```python
from build123d import *

# Parameters (mm, degrees)
SKETCH_W        = 105
SKETCH_H        = 110
PAD_DEPTH       = 7.5
SKETCH001_R     = 1.25
POCKET_DEPTH    = 8
SKETCH002_R     = 3
POCKET001_DEPTH = 6
SKETCH003_W     = 85
SKETCH003_H     = 110
SKETCH003_W_2   = 81
SKETCH003_H_2   = 106
PAD001_DEPTH    = 57
SKETCH004_R     = 3.29
POCKET002_DEPTH = 6
SKETCH005_W     = 10
SKETCH005_H     = 110
POCKET003_DEPTH = 4
SKETCH006_W     = 10
SKETCH006_H     = 110
POCKET004_DEPTH = 4
SKETCH007_R     = 2.5
POCKET005_DEPTH = 5
SKETCH008_W     = 16
SKETCH008_H     = 16
POCKET006_DEPTH = 5
SKETCH009_R     = 1.25
SKETCH009_W     = 3.5
SKETCH009_H     = 7.5
POCKET007_DEPTH = 5


with BuildPart() as part:
    # Sketch → Pad (new body)
    with BuildSketch(Plane.XY):
        Rectangle(SKETCH_W, SKETCH_H)
    extrude(amount=PAD_DEPTH)

    # Sketch001 (on Face6 of Pad) → Pocket (cut)
    with BuildSketch(Plane.XY.offset(7.5)):
        with Locations((-33.5, 41.5)):
            Circle(SKETCH001_R)
        with Locations((15.5, 41.5)):
            Circle(SKETCH001_R)
        with Locations((-33.5, -16.5)):
            Circle(SKETCH001_R)
        with Locations((15.5, -16.5)):
            Circle(SKETCH001_R)
    extrude(amount=-POCKET_DEPTH, mode=Mode.SUBTRACT)

    # Sketch002 (on Face4 of Pocket) → Pocket001 (cut)
    with BuildSketch(Plane(origin=(0, 0, 0), x_dir=(1, 0, 0), z_dir=(0, 0, -1))):
        with Locations((-33.5, 16.5)):
            Circle(SKETCH002_R)
        with Locations((15.5, 16.5)):
            Circle(SKETCH002_R)
        with Locations((-33.5, -41.5)):
            Circle(SKETCH002_R)
        with Locations((15.5, -41.5)):
            Circle(SKETCH002_R)
    extrude(amount=-POCKET001_DEPTH, mode=Mode.SUBTRACT)

    # Sketch003 (on Face5 of Pocket001) → Pad001 (join)
    with BuildSketch(Plane.XY.offset(7.5)):
        Rectangle(SKETCH003_W, SKETCH003_H)
        Rectangle(SKETCH003_W_2, SKETCH003_H_2, mode=Mode.SUBTRACT)
    extrude(amount=PAD001_DEPTH)

    # Sketch004 (on Face29 of Pad001) → Pocket002 (cut)
    with BuildSketch(Plane.XY.offset(7.5)):
        with Locations((-36.21, 48.71)):
            Circle(SKETCH004_R)
        with Locations((36.21, 48.71)):
            Circle(SKETCH004_R)
        with Locations((-36.21, -48.71)):
            Circle(SKETCH004_R)
        with Locations((36.21, -48.71)):
            Circle(SKETCH004_R)
    extrude(amount=-POCKET002_DEPTH, mode=Mode.SUBTRACT)

    # Sketch005 (on Face5 of Pocket002) → Pocket003 (cut)
    with BuildSketch(Plane.XY.offset(7.5)):
        with Locations((-47.5, 0)):
            Rectangle(SKETCH005_W, SKETCH005_H)
    extrude(amount=-POCKET003_DEPTH, mode=Mode.SUBTRACT)

    # Sketch006 (on Face4 of Pocket003) → Pocket004 (cut)
    with BuildSketch(Plane.XY.offset(7.5)):
        with Locations((47.5, 0)):
            Rectangle(SKETCH006_W, SKETCH006_H)
    extrude(amount=-POCKET004_DEPTH, mode=Mode.SUBTRACT)

    # Sketch007 (on Face8 of Pocket004) → Pocket005 (cut)
    with BuildSketch(Plane.XY.offset(3.5)):
        with Locations((-47.5, 45)):
            Circle(SKETCH007_R)
        with Locations((-47.5, 0)):
            Circle(SKETCH007_R)
        with Locations((-47.5, -45)):
            Circle(SKETCH007_R)
        with Locations((47.5, 45)):
            Circle(SKETCH007_R)
        with Locations((47.5, 0)):
            Circle(SKETCH007_R)
        with Locations((47.5, -45)):
            Circle(SKETCH007_R)
    extrude(amount=-POCKET005_DEPTH, mode=Mode.SUBTRACT)

    # Sketch008 (on Face24 of Pocket005) → Pocket006 (cut)
    with BuildSketch(Plane.XZ.offset(55)):
        with Locations((-8, 27)):
            Rectangle(SKETCH008_W, SKETCH008_H)
    extrude(amount=-POCKET006_DEPTH, mode=Mode.SUBTRACT)

    # Sketch009 (on Face21 of Pocket006) → Pocket007 (cut)
    with BuildSketch(Plane.YZ.offset(42.5)):
        with Locations((-10.15, 56.5)):
            Circle(SKETCH009_R)
        with Locations((10.15, 56.5)):
            Circle(SKETCH009_R)
        with Locations((-10.15, 44.33)):
            Circle(SKETCH009_R)
        with Locations((10.15, 44.33)):
            Circle(SKETCH009_R)
        with Locations((16.9, 50.75)):
            Rectangle(SKETCH009_W, SKETCH009_H)
    extrude(amount=-POCKET007_DEPTH, mode=Mode.SUBTRACT)


solid = part.part
```
Part model, mm, in its own coordinate system. A direction names the side the tool comes from. Round coordinates to 2 decimals unless told otherwise and drop trailing zeros. Order: outer loops, then holes, each group sorted by start corner. A loop starts at its lowest first (then second) coordinate and runs counter-clockwise, first axis right, second up. Notation, with made-up numbers: M 40,-20 L 58,-20 A32 cw 58,12 Z; hole C 46,14 d6. An arc over 180 degrees is marked long. Put each result on its own line as item: value. Start each with the question number.
1. Slice it at A-A on y = -41. List the corners of the cut face in (x, z).
2. Tool access for faces 5 (the face through (-36.5, -16.6, 3)), 6 (the face through (-42.5, -1, 34)), 7 (the face through (33.6, -50.71, 4.54)): list every direction of +Z, -Z, +X, -X, +Y, -Y with a clear straight run to the whole face (end or side of a thin tool).
3. Slice it at B-B on z = 26. List the corners of the cut face in (x, y), then the cut area to 3 significant figures.
4. Slice it at D-D on x = 27. List the corners of the cut face in (y, z), then the cut area to 3 significant figures.
5. Drop flat-ended pins along their axis: pin 1 (2 mm diameter, centred on x = -33.5, y = -16.5, fed in from +Z); pin 2 (3 mm diameter, centred on y = -8.5, z = 8.5, fed in from -X); pin 3 (6.5 mm diameter, centred on x = 47.5, y = -45, fed in from +Z). Give the stop position or say it passes through.
6. Slice it at C-C on y = 0. List the corners of the cut face in (x, z), then the cut area to 4 significant figures.
7. Drill centre lines: probe 1 along X at (y, z) = (41.5, 3.8); probe 2 along Z at (x, y) = (41.65, 10.15); probe 3 along X at (y, z) = (48, 50.5). Where is each one in solid material? Low to high. Write a range as [from, to].
8. Two-plate mould, pull along X, no slides. Class faces 1 (the face through (-1, 1, 0)), 2 (the face through (42.5, -1, 34)), 3 (the face through (-34.441, 51.484, 4.542)), 4 (the face through (15.34, -15.26, 6.76)): +X half, -X half, draft (parallel to the pull), parting line (faces both ways), or undercut.
Findings:
1. outline: M -52.5,0 L 52.5,0 L 52.5,3.5 L 42.5,3.5 L 42.5,64.5 L 40.5,64.5 L 40.5,7.5 L -40.5,7.5 L -40.5,64.5 L -42.5,64.5 L -42.5,3.5 L -52.5,3.5 Z
2. face 5: -Z
2. face 6: +Z, -X, +Y, -Y
2. face 7: +Z
3. outline: M -42.5,-55 L -16,-55 L -16,-53 L -40.5,-53 L -40.5,53 L 40.5,53 L 40.5,-53 L 0,-53 L 0,-55 L 42.5,-55 L 42.5,55 L -42.5,55 Z
3. area: 732 mm2
4. outline: M -55,0 L 55,0 L 55,64.5 L 53,64.5 L 53,7.5 L -53,7.5 L -53,64.5 L -55,64.5 Z
4. area: 1,050 mm2
5. pin 1: through
5. pin 2: x = -42.5
5. pin 3: z = 3.5
6. outline: M -52.5,0 L -50,0 L -50,3.5 L -52.5,3.5 Z; M -45,0 L 45,0 L 45,3.5 L 42.5,3.5 L 42.5,64.5 L 40.5,64.5 L 40.5,7.5 L -40.5,7.5 L -40.5,64.5 L -42.5,64.5 L -42.5,3.5 L -45,3.5 Z; M 50,0 L 52.5,0 L 52.5,3.5 L 50,3.5 Z
6. area: 900.5 mm2
7. probe 1: [-42.5, -36.5], [-30.5, 12.5], [18.5, 42.5]
7. probe 2: [0, 43.08], [45.58, 55.25], [57.75, 64.5]
7. probe 3: [-42.5, -40.5], [40.5, 42.5]
8. face 1: draft
8. face 2: +X half
8. face 3: undercut
8. face 4: undercut
